Design review of the part built by this model. Coordinates are the model's own, in mm. A direction names the side the tool comes from. Coordinates: 2 decimals unless noted, no trailing zeros. Write each loop counter-clockwise with the first axis right and the second up, starting at its lowest first coordinate (ties: lowest second). Pieces come first, ordered by that corner, then holes. Notation, with made-up numbers: (25.25, 16) - (29.25, 16) arc R12 cw to (29.25, 30) - close; hole circle Ø5 at (88, 59). An arc over 180 degrees is marked (long way). Answer as a JSON object with one key per item and string values.
```python
from build123d import *

# Parameters (mm, degrees)
F3_DEPTH = 5
F4_SIZE  = 0.8


with BuildPart() as f1:
    # F0 (on Front) → F1 (revolve)
    with BuildSketch(Plane.XZ):
        Polygon((42.6336441377, -121.3015150939), (39.937491715, -122.8581394209), (39.937491715, -124.3015150939), (63.437491715, -124.3015150939), (63.437491715, -120.3015150939), (48.0148419841, -120.3015150939), (47.437491715, -121.3015150939), align=None)
    revolve(axis=Axis((51.687491715, 0, -124.3015150939), (-1, 0, 0)))

    # F2 (on face) → F3 (cut)
    with BuildSketch(Plane.YZ.offset(63.437491715)):
        Polygon((2.7500788948, -123.423791102), (0.6149081729, -121.4810149127), (-2.1351707219, -122.3587389045), (-2.7500788948, -125.1792390858), (-0.6149081729, -127.1220152751), (2.1351707219, -126.2442912832), align=None)
    extrude(amount=-F3_DEPTH, mode=Mode.SUBTRACT)

    # F4
    f4_edges = [f1.edges().sort_by_distance(p)[0] for p in [
        (63.437492, 0, -128.301515),
    ]]
    chamfer(f4_edges, length=F4_SIZE)


solid = f1.part
```
(1) To check wall thickness, follow line 1 (Y direction, x = 43.5, z = -124.25); line 2 (Y direction, x = 53, z = -124.5); line 3 (Z direction, x = 60.25, y = 1). State the ranges of each line that lie inside material, in increasing order. Write a range as from..to.
Solved:
{"line 1": "y = -3..3", "line 2": "y = -4..4", "line 3": "z = -128.17..-126.61, -121.83..-120.43"}
(2) For pin 1 (3 mm diameter, centred on y = -0.5, z = -123.5, fed in from +X); pin 2 (1 mm diameter, centred on x = 48, y = 2.5, fed in from +Z), all flat-tipped, find the tip position at first contact; note any pin that passes through.
Solved:
{"pin 1": "stops at x = 58.44", "pin 2": "stops at z = -120.84"}
(3) Take a section at C-C, the plane x = 44.5. Write out the cut boundary in (y, z), and give its area (3 significant figures).
Solved:
{"outline": "circle Ø6 at (0, -124.3)", "area": "28.3 mm^2"}
(4) Tool access review of faces 4 (the face through (45, 0.9, -121.44)), 5 (the face through (39.937, 0, -124)), 6 (the face through (60.972, -1.697, -126.137)): name each direction out of +Z, -Z, +X, -X, +Y, -Y from which nothing blocks a thin tool from reaching the whole face with its end or side.
Solved:
{"face 4": "-X", "face 5": "+Z, -Z, -X, +Y, -Y", "face 6": "+X"}
(5) Take a section at A-A, the plane x = 55. Write out the cut boundary in (y, z).
Solved:
{"outline": "circle Ø8 at (0, -124.3)"}
(6) The part is to be moulded in two halves that separate along Z. For faces 1 (the face through (63.437, 2, -122)), 2 (the face through (60.97, 1.7, -122.47)), 3 (the face through (55.224, 0.176, -128.298)), say which applies: pulls with the +Z half, pulls with the -Z half, needs draft (parallel to the pull), parting line crosses it, or undercut.
Solved:
{"face 1": "needs draft", "face 2": "undercut", "face 3": "parting line crosses it"}
(7) Take a section at B-B, the plane y = 0. Write out the cut boundary in (x, z), and give its area (3 significant figures).
Solved:
{"outline": "(39.94, -125.74) - (42.63, -127.3) - (47.44, -127.3) - (48.01, -128.3) - (62.64, -128.3) - (63.44, -127.5) - (63.44, -126.93) - (58.44, -126.93) - (58.44, -121.68) - (63.44, -121.68) - (63.44, -121.1) - (62.64, -120.3) - (48.01, -120.3) - (47.44, -121.3) - (42.63, -121.3) - (39.94, -122.86) - close", "area": "141 mm^2"}
